from build123d import *

# Parameters (mm, degrees)
F0_R     = 10
F0_R_2   = 4
F1_DEPTH = 3
F3_DEPTH = 25
F4_DEPTH = 3


# Not quite as in the source:
# - a feature names something its author has since deleted; it is built from what else it names


with BuildPart() as f1:
    # F0 (on Top) → F1 (new body)
    with BuildSketch(Plane.XY):
        with Locations((0, -55)):
            Circle(F0_R)
        with Locations((0, -55)):
            Circle(F0_R_2, mode=Mode.SUBTRACT)
    extrude(amount=-F1_DEPTH)

    # F2 (on face) → F3 (cut)
    with BuildSketch(Plane.XY):
        with BuildLine():
            ThreePointArc((6.918967171, -54.711004694), (6.9234916285, -54.8554708664), (6.925, -55))
            ThreePointArc((6.925, -55), (6.9091405252, -55.4684038892), (6.8616347427, -55.9346623229))
            Line((6.8616347427, -55.9346623229), (7.7608112736, -56.2391925528))
            Line((7.7608112736, -56.2391925528), (8.4266122732, -56.5844591584))
            Line((8.4266122732, -56.5844591584), (9.0325271812, -57.0264626926))
            Line((9.0325271812, -57.0264626926), (9.5646125465, -57.5550316702))
            Line((9.5646125465, -57.5550316702), (9.3682753061, -58.2008464176))
            Line((9.3682753061, -58.2008464176), (8.6320298332, -58.3438240508))
            Line((8.6320298332, -58.3438240508), (7.8826287699, -58.373791473))
            Line((7.8826287699, -58.373791473), (7.1373175032, -58.2900590671))
            Line((7.1373175032, -58.2900590671), (6.2207936805, -58.0425895196))
            ThreePointArc((6.2207936805, -58.0425895196), (5.9273034064, -58.5808796864), (5.5873528695, -59.0911016746))
            Line((5.5873528695, -59.0911016746), (6.2328020031, -59.7872715608))
            Line((6.2328020031, -59.7872715608), (6.6536597658, -60.4080603684))
            Line((6.6536597658, -60.4080603684), (6.9757740672, -61.0853656001))
            Line((6.9757740672, -61.0853656001), (7.1917323401, -61.8036009545))
            Line((7.1917323401, -61.8036009545), (6.7114037747, -62.2778471661))
            Line((6.7114037747, -62.2778471661), (5.9959787098, -62.0527539043))
            Line((5.9959787098, -62.0527539043), (5.322833198, -61.722034809))
            Line((5.322833198, -61.722034809), (4.7074578164, -61.2933004628))
            Line((4.7074578164, -61.2933004628), (4.0195694603, -60.6390323951))
            ThreePointArc((4.0195694603, -60.6390323951), (3.5050568866, -60.9724535345), (2.9630704597, -61.2590605087))
            Line((2.9630704597, -61.2590605087), (3.1988405858, -62.1786634351))
            Line((3.1988405858, -62.1786634351), (3.2730686388, -62.9249811932))
            Line((3.2730686388, -62.9249811932), (3.2335539791, -63.673939531))
            Line((3.2335539791, -63.673939531), (3.0812059272, -64.4083032495))
            Line((3.0812059272, -64.4083032495), (2.4329416781, -64.5963948851))
            Line((2.4329416781, -64.5963948851), (1.9111960197, -64.0576171313))
            Line((1.9111960197, -64.0576171313), (1.476949591, -63.4461189391))
            Line((1.476949591, -63.4461189391), (1.1401953689, -62.7759722433))
            Line((1.1401953689, -62.7759722433), (0.8471481357, -61.8729880719))
            ThreePointArc((0.8471481357, -61.8729880719), (0.2359283481, -61.9209799028), (-0.3771407279, -61.9147226894))
            Line((-0.3771407279, -61.9147226894), (-0.6080157262, -62.8355667749))
            Line((-0.6080157262, -62.8355667749), (-0.898352157, -63.5270902792))
            Line((-0.898352157, -63.5270902792), (-1.2899483564, -64.1667405091))
            Line((-1.2899483564, -64.1667405091), (-1.773792824, -64.7397976887))
            Line((-1.773792824, -64.7397976887), (-2.4333609662, -64.5962885747))
            Line((-2.4333609662, -64.5962885747), (-2.6353644947, -63.8740042993))
            Line((-2.6353644947, -63.8740042993), (-2.7257904358, -63.1294754891))
            Line((-2.7257904358, -63.1294754891), (-2.7025578872, -62.3798354097))
            Line((-2.7025578872, -62.3798354097), (-2.5299587465, -61.4463116385))
            ThreePointArc((-2.5299587465, -61.4463116385), (-3.0902045366, -61.1972785093), (-3.6262282301, -60.8996689588))
            Line((-3.6262282301, -60.8996689588), (-4.267964983, -61.5992624369))
            Line((-4.267964983, -61.5992624369), (-4.852715623, -62.0689077169))
            Line((-4.852715623, -62.0689077169), (-5.5017769863, -62.4446993436))
            Line((-5.5017769863, -62.4446993436), (-6.2002127258, -62.7179895151))
            Line((-6.2002127258, -62.7179895151), (-6.2293167628, -62.8227624704))
            ThreePointArc((-6.2293167628, -62.8227624704), (4.3420520709, -64.0081398643), (10, -55))
            ThreePointArc((10, -55), (8.9702732091, -50.5802490393), (6.093160289, -47.0707252733))
            Line((6.093160289, -47.0707252733), (4.5292177041, -49.7615067062))
            Line((4.5292177041, -49.7615067062), (5.2752674988, -49.1744234085))
            Line((5.2752674988, -49.1744234085), (5.9280342708, -48.8051057384))
            Line((5.9280342708, -48.8051057384), (6.6291535281, -48.5387755166))
            Line((6.6291535281, -48.5387755166), (7.3624909556, -48.3815615944))
            Line((7.3624909556, -48.3815615944), (7.7963725922, -48.8986415935))
            Line((7.7963725922, -48.8986415935), (7.5142043948, -49.5935380667))
            Line((7.5142043948, -49.5935380667), (7.1301722462, -50.2377579894))
            Line((7.1301722462, -50.2377579894), (6.653113581, -50.8164764269))
            Line((6.653113581, -50.8164764269), (5.9453992104, -51.4492461041))
            ThreePointArc((5.9453992104, -51.4492461041), (6.2361540084, -51.9890187341), (6.4780276654, -52.552392481))
            Line((6.4780276654, -52.552392481), (7.4136750809, -52.3917033141))
            Line((7.4136750809, -52.3917033141), (8.1635503464, -52.3780253684))
            Line((8.1635503464, -52.3780253684), (8.9068663995, -52.4779315504))
            Line((8.9068663995, -52.4779315504), (9.6265178829, -52.6891227965))
            Line((9.6265178829, -52.6891227965), (9.7616104212, -53.350466131))
            Line((9.7616104212, -53.350466131), (9.1824341074, -53.8269688042))
            Line((9.1824341074, -53.8269688042), (8.5378456767, -54.2103820995))
            Line((8.5378456767, -54.2103820995), (7.8426785438, -54.4918828231))
            Line((7.8426785438, -54.4918828231), (6.918967171, -54.711004694))
        make_face()
    extrude(amount=-F3_DEPTH, mode=Mode.SUBTRACT)

    # F0 (on Top) → F4 (join)
    with BuildSketch(Plane.XY):
        with Locations((0, -55)):
            Circle(F0_R)
        with Locations((0, -55)):
            Circle(F0_R_2, mode=Mode.SUBTRACT)
    extrude(amount=F4_DEPTH)


solid = f1.part
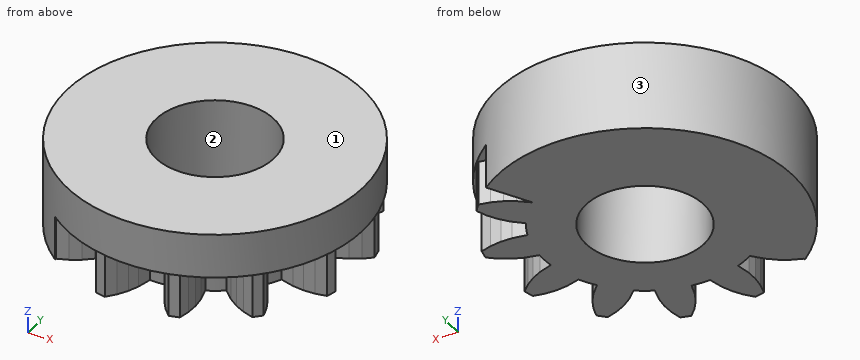
Work out the finished part from the listing and answer in its coordinate system (mm). Face numbers are marked on the shaded views. Round coordinates to 2 decimals unless told otherwise and drop trailing zeros. Write each loop counter-clockwise with the first axis right and the second up, starting at its lowest first coordinate (ties: lowest second). Pieces come first, ordered by that corner, then holes. Notation, with made-up numbers: (46, 36.5) - (66, 36.5) arc R27 ccw to (66, 53.5) - close; hole circle Ø6 at (-30.75, 84). An arc over 180 degrees is marked (long way). Answer in a Markdown table with one row per item. Add a question column.
1. Given pin 1 (3 mm diameter, centred on x = -4.5, z = 0, fed in from +Y); pin 2 (6.5 mm diameter, centred on x = 0, y = -55, fed in from +Z); pin 3 (1 mm diameter, centred on x = -6.5, z = 1.5, fed in from +Y), each flat-ended and moving along its own axis, determine where each tip first touches the part or whether it passes through.
2. Find the intervals of material crossed by line 1 along Y through (x, z) = (0, 0.7); line 2 along X through (y, z) = (-61.75, -2.7); line 3 along Y through (x, z) = (6.25, -0.9), in increasing order. Write a range as from..to.
3. A cutting plane is placed at A-A, the plane x = 0. Determine the outline of the cut face in (y, z) (3 decimals), and give its area (3 significant figures).
4. A cutting plane is placed at B-B, the plane y = -59.5. Determine the outline of the cut face in (x, z), and give its area (3 significant figures).
5. The mould has two halves that part along Y. Classify the marked faces 1, 2 and 3: +Y half, -Y half, draft (parallel to the pull), parting line (faces both ways), or undercut.
Worked out:
| question | item | result |
|---|---|---|
| 1 | pin 1 | y = -45.46 |
| 1 | pin 2 | through |
| 1 | pin 3 | y = -47 |
| 2 | line 1 | -65..-59, -51..-45 |
| 2 | line 2 | -7.38..-4.46, -2.59..3.09, 5.38..7.18 |
| 2 | line 3 | -62.13..-59.81, -58.05..-52.02, -51.18..-48.68 |
| 3 | outline | (-65, 0) - (-61.925, 0) - (-61.925, -3) - (-59, -3) - (-59, 3) - (-65, 3) - close; (-51, -3) - (-45, -3) - (-45, 3) - (-51, 3) - close |
| 3 | area | 62.8 mm^2 |
| 4 | outline | (-8.93, -3) - (5.97, -3) - (5.97, 0) - (8.93, 0) - (8.93, 3) - (-8.93, 3) - close |
| 4 | area | 98.3 mm^2 |
| 5 | face 1 | draft |
| 5 | face 2 | undercut |
| 5 | face 3 | parting line |
